Could you check a few things on this model? Use its own coordinates, in mm. A direction names the side the tool comes from. Give positions to 0.01 mm unless a question says otherwise; leave off trailing zeros. Write each loop counter-clockwise with the first axis right and the second up, starting at its lowest first coordinate (ties: lowest second). Pieces come first, ordered by that corner, then holes. Notation, with made-up numbers: M 72.25,34.25 L 90.25,34.25 A18 cw 90.25,63.25 Z; hole C 41,42.25 d11. An arc over 180 degrees is marked long. Use one line per item in the form item = value.
from build123d import *

# Parameters (mm, degrees)
SKETCH_1_W             = 25
SKETCH_1_H             = 25
SKETCH_1_W_2           = 19
SKETCH_1_H_2           = 19
EXTRUDE_1_DEPTH        = 754.5
HOLE_WIZARD_6_0_6_1_D  = 6
CUT_EXTRUDE_1_REACH    = 757.328
SKETCH_5_R             = 6
PATTERN_LINEAR_1_COUNT = 2
PATTERN_LINEAR_1_PITCH = 684.3


with BuildPart() as part:
    # Sketch 1 → Extrude 1 (new body)
    with BuildSketch(Plane.XY):
        with Locations((12.5, -12.5)):
            Rectangle(SKETCH_1_W, SKETCH_1_H)
        with Locations((12.5, -12.5)):
            Rectangle(SKETCH_1_W_2, SKETCH_1_H_2, mode=Mode.SUBTRACT)
    extrude(amount=EXTRUDE_1_DEPTH)

    # Hole Wizard 6.0 _6_ _1 (through all)
    with Locations(Plane(origin=(25, 0, 0), x_dir=(0, 0, -1), z_dir=(1, 0, 0))):
        with Locations((-705.5, -12.5), (-733.5, -12.5)):
            hole_wizard_6_0_6_1 = Hole(HOLE_WIZARD_6_0_6_1_D / 2)

    # Sketch 5 → Cut-Extrude 1 (cut, up to next)
    with BuildSketch(Plane.ZY, mode=Mode.PRIVATE) as cut_extrude_1_sk1:
        with Locations(Location((705.5, -12.5, 0), (0, 0, 270))):
            Circle(SKETCH_5_R)
    cut_extrude_1_tool1 = extrude(cut_extrude_1_sk1.sketch, amount=-CUT_EXTRUDE_1_REACH, mode=Mode.PRIVATE) & part.part
    # Sketch 5 → Cut-Extrude 1 (cut, up to next)
    with BuildSketch(Plane.ZY, mode=Mode.PRIVATE) as cut_extrude_1_sk2:
        with Locations(Location((733.5, -12.5, 0), (0, 0, 270))):
            Circle(SKETCH_5_R)
    cut_extrude_1_tool2 = extrude(cut_extrude_1_sk2.sketch, amount=-CUT_EXTRUDE_1_REACH, mode=Mode.PRIVATE) & part.part
    cut_extrude_1_1 = cut_extrude_1_tool1.solids().sort_by_distance((0, -12.5, 705.5))[0]
    add(cut_extrude_1_1, mode=Mode.SUBTRACT)
    cut_extrude_1_2 = cut_extrude_1_tool2.solids().sort_by_distance((0, -12.5, 733.5))[0]
    add(cut_extrude_1_2, mode=Mode.SUBTRACT)
    cut_extrude_1 = cut_extrude_1_1 + cut_extrude_1_2  # Cut-Extrude 1 as one shape, for the pattern or mirror that repeats it

    # Pattern Linear 1: Hole Wizard 6.0 _6_ _1, Cut-Extrude 1 ×2
    with Locations(*[(0, 0, -i * PATTERN_LINEAR_1_PITCH) for i in range(1, PATTERN_LINEAR_1_COUNT)]):
        add(hole_wizard_6_0_6_1, mode=Mode.SUBTRACT)
        add(cut_extrude_1, mode=Mode.SUBTRACT)


solid = part.part
1) Thinking about a two-plate mould opening in Z: for faces 4 (the cylindrical face through (1.48, -11.72, 711.45)), 5 (the flat face through (23, -12, 0)), 6 (the flat face through (23, -12, 754.5)), which applies, released by +Z, released by -Z, zero draft, split by the parting line, or undercut?
Checked values:
face_4 = undercut
face_5 = released by -Z
face_6 = released by +Z
2) I want a section at B-B, the plane z = 458. Please give me the cut outline in (x, y), plus the area to 3 significant figures.
Checked values:
outline = M 0,-25 L 25,-25 L 25,0 L 0,0 Z; hole M 3,-22 L 22,-22 L 22,-3 L 3,-3 Z
area = 264 mm2
3) For pin 1 Ø9.5 at (y, z) = (-12.5, 733.5) entering from -X, with a flat end and sliding along its axis, tell me the tip position at first contact or that it passes through.
Checked values:
pin_1 = 22
4) I want a section at A-A, the plane x = 13.25. Please give me the cut outline in (y, z), plus the area to 3 significant figures.
Checked values:
outline = M -25,0 L -22,0 L -22,754.5 L -25,754.5 Z; M -3,0 L 0,0 L 0,754.5 L -3,754.5 Z
area = 4,530 mm2
5) If I drill on L1, parallel to Z at x = 2.1, y = -12.5; L2, parallel to Y at x = 17.75, z = 250; L3, parallel to X at y = -17.25, z = 607, over which ranges is the centre line in solid material (lowest first)?
Checked values:
L1 = 0 to 15.2, 27.2 to 43.2, 55.2 to 699.5, 711.5 to 727.5, 739.5 to 754.5
L2 = -25 to -22, -3 to 0
L3 = 0 to 3, 22 to 25
6) For faces 1 (the flat face through (0, -13, 372)), 2 (the flat face through (12, -3, 372)), 3 (the cylindrical face through (1.48, -18.04, 18.9)), which set-ups out of +Z, -Z, +X, -X, +Y, -Y let a thin tool reach every point of the face, with its end or its side?
Checked values:
face_1 = +Z, -Z, -X, +Y, -Y
face_2 = +Z, -Z
face_3 = -X
